```python
from build123d import *


with BuildPart() as part:
    # Skizze1 → Rotation1 (revolve)
    with BuildSketch(Plane.XY, mode=Mode.PRIVATE) as rotation1_sk:
        Polygon((36.6, 0), (46.1, 0), (46.1, 0.7), (47.5, 0.7), (47.5, 3.3), (46.1, 3.3), (46.1, 4), (36.6, 4), (36.6, 3.3), (35, 3.3), (35, 0.7), (36.6, 0.7), align=None)
    revolve(rotation1_sk.sketch.rotate(Axis((0, 0, 0), (0, 1, 0)), 90), axis=Axis((0, 0, 0), (0, 1, 0)))


solid = part.part
```
For this review, take the finished solid that the model builds, in its own axes (mm). A direction names the side the tool comes from. Give positions to 0.01 mm unless a question says otherwise; leave off trailing zeros. Write each loop counter-clockwise with the first axis right and the second up, starting at its lowest first coordinate (ties: lowest second). Pieces come first, ordered by that corner, then holes.
Item 1: Wall thickness on probe 1 along X at (y, z) = (2.1, 0); probe 2 along X at (y, z) = (3.6, 0); probe 3 along Z at (x, y) = (-7, 3.8): over which ranges is each line inside the solid? List them lowest first.
Item 2: Machinability: for faces 4 (the face through (30, 3.3, -19)), 5 (the face through (-30.86, 0.35, -19.68)), 6 (the face through (46.37, 2.02, 10.3)), which of the approach directions +Z, -Z, +X, -X, +Y, -Y give a long, thin tool a straight path to every point of the face, cutting with its end or side? Answer none if there is none.
Item 3: Insertion check: P1, Ø1.5, axis at x = -6.5, y = 2, coming from the -Z side; P2, Ø2, axis at y = 1, z = 24.5, coming from the +X side; P3, Ø1, axis at x = 19, y = 2.5, coming from the -Z side. Each pin has a flat end and moves straight along its axis. Give the tip position at first contact, or say it passes through.
Item 4: Take a section at B-B (z = 0). Give the boundary of the cut face in (x, y).
Item 5: The part is to be moulded in two halves that separate along X. For faces 1 (the face through (-24, 4, 28)), 2 (the face through (-30.86, 3.65, -19.68)), 3 (the face through (-13.85, 0.35, -43.97)), say which applies: +X half, -X half, draft (parallel to the pull), parting line (faces both ways), or undercut.
Item 6: Take a section at C-C (y = 1.85). Give the boundary of the cut face in (x, z), and give its area (3 significant figures).
Item 7: Take a section at A-A (x = 0). Give the boundary of the cut face in (y, z).
Established:
1. probe 1: x = -47.5 to -35, 35 to 47.5
1. probe 2: x = -46.1 to -36.6, 36.6 to 46.1
1. probe 3: z = -45.57 to -35.92, 35.92 to 45.57
2. face 4: +Y
2. face 5: -Y
2. face 6: +Y, -Y
3. P1: stops at z = -47.15
3. P2: stops at x = 41.28
3. P3: stops at z = -43.75
4. outline: (-47.5, 0.7) - (-46.1, 0.7) - (-46.1, 0) - (-36.6, 0) - (-36.6, 0.7) - (-35, 0.7) - (-35, 3.3) - (-36.6, 3.3) - (-36.6, 4) - (-46.1, 4) - (-46.1, 3.3) - (-47.5, 3.3) - close; (35, 0.7) - (36.6, 0.7) - (36.6, 0) - (46.1, 0) - (46.1, 0.7) - (47.5, 0.7) - (47.5, 3.3) - (46.1, 3.3) - (46.1, 4) - (36.6, 4) - (36.6, 3.3) - (35, 3.3) - close
5. face 1: draft
5. face 2: undercut
5. face 3: parting line
6. outline: circle Ø95 at (0, 0); hole circle Ø70 at (0, 0)
6. area: 3,240 mm2
7. outline: (0, -46.1) - (0.7, -46.1) - (0.7, -47.5) - (3.3, -47.5) - (3.3, -46.1) - (4, -46.1) - (4, -36.6) - (3.3, -36.6) - (3.3, -35) - (0.7, -35) - (0.7, -36.6) - (0, -36.6) - close; (0, 36.6) - (0.7, 36.6) - (0.7, 35) - (3.3, 35) - (3.3, 36.6) - (4, 36.6) - (4, 46.1) - (3.3, 46.1) - (3.3, 47.5) - (0.7, 47.5) - (0.7, 46.1) - (0, 46.1) - close
